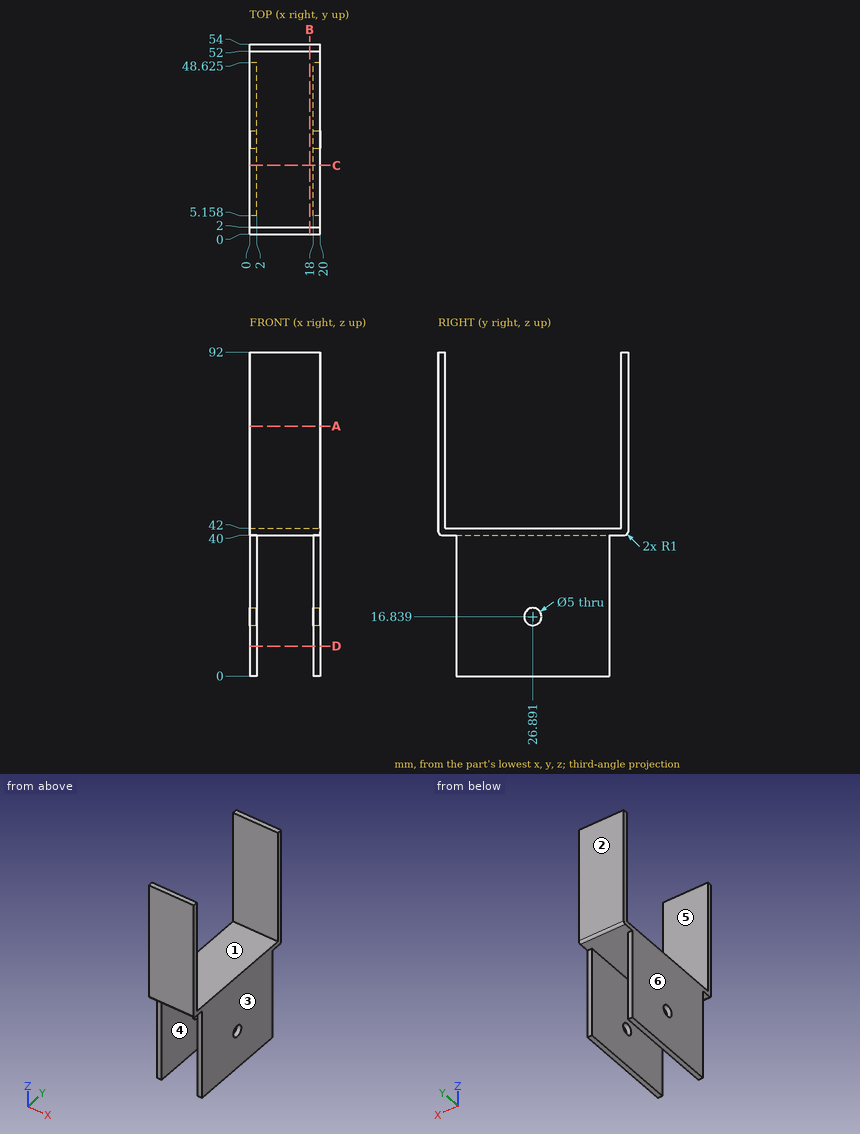
Job drawing, mm, ordinate dimensions from the low corner. One solid piece. A direction names the side the tool comes from. Coordinates: 2 decimals unless noted, no trailing zeros. Write each loop counter-clockwise with the first axis right and the second up, starting at its lowest first coordinate (ties: lowest second). Pieces come first, ordered by that corner, then holes.
Item 1: Slice it at B-B (x = 17). Write the cut outline in (y, z).
Item 2: Which spindle directions (+Z, -Z, +X, -X, +Y, -Y) get a long thin tool onto all of the face, cutting with end or side? Do the marked faces 4, 5 and 6. Say none if no direction does.
Item 3: Slice it at A-A (z = 71). Write the cut outline in (x, y).
Item 4: Slice it at D-D (z = 8.5). Write the cut outline in (x, y) (1 decimal).
Item 5: Pin check, flat tips, straight feed: pin 1 (1.6 mm diameter, centred on x = 0.5, z = 17.5, fed in from +Y) (1 decimal); pin 2 (5 mm diameter, centred on x = 7, y = 47.5, fed in from +Z); pin 3 (1.6 mm diameter, centred on x = 1, z = 10.5, fed in from -Y); pin 4 (1 mm diameter, centred on x = 16, z = 11.5, fed in from +Y). Stop position of each tip, or through.
Item 6: Mould opens along Y. For the marked faces 1, 2 and 3 say: released by +Y, released by -Y, zero draft, split by the parting line, or undercut.
Item 7: Probe line 1 (Y direction, x = 12.5, z = 42.5); line 2 (X direction, y = 22, z = 38); line 3 (Y direction, x = 1.5, z = 20) (1 decimal). List the from-to ranges inside material, lowest first.
Item 8: Slice it at C-C (y = 19.5). Write the cut outline in (x, z).
Results found:
1. outline: (0, 41) arc R1 ccw to (1, 40) - (53, 40) arc R1 ccw to (54, 41) - (54, 92) - (52, 92) - (52, 42) - (2, 42) - (2, 92) - (0, 92) - close
2. face 4: -Z, +Y, -Y
2. face 5: +Z, +X, -X
2. face 6: +Z, -Z, -X, +Y, -Y
3. outline: (0, 0) - (20, 0) - (20, 2) - (0, 2) - close; (0, 52) - (20, 52) - (20, 54) - (0, 54) - close
4. outline: (0, 5.2) - (2, 5.2) - (2, 48.6) - (0, 48.6) - close; (18, 5.2) - (20, 5.2) - (20, 48.6) - (18, 48.6) - close
5. pin 1: stops at y = 48.6
5. pin 2: stops at z = 42
5. pin 3: stops at y = 5.16
5. pin 4: passes through
6. face 1: undercut
6. face 2: released by +Y
6. face 3: zero draft
7. line 1: y = 0 to 2, 52 to 54
7. line 2: x = 0 to 2, 18 to 20
7. line 3: y = 5.2 to 48.6
8. outline: (0, 0) - (2, 0) - (2, 40) - (18, 40) - (18, 0) - (20, 0) - (20, 42) - (0, 42) - close
